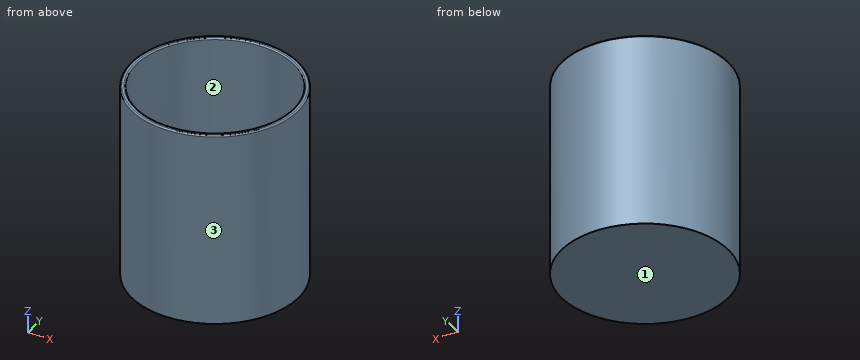
```python
from build123d import *

# Parameters (mm, degrees)
F0_R     = 30
F1_DEPTH = 70
F2_T     = -1.75
F3_R     = 0.5


with BuildPart() as f1:
    # F0 (on Top) → F1 (new body)
    with BuildSketch(Plane.XY):
        Circle(F0_R)
    extrude(amount=F1_DEPTH)

    # F2
    f2_openings = [f1.faces().sort_by_distance(p)[0] for p in [
        (0, 0, 70),
    ]]
    offset(amount=F2_T, openings=f2_openings)

    # F3
    f3_edges = [f1.edges().sort_by_distance(p)[0] for p in [
        (-30, 0, 70),
        (-28.25, 0, 70),
    ]]
    fillet(f3_edges, radius=F3_R)


solid = f1.part
```
CAD build for the part. Positions are in the model's coordinates, mm. Face numbers are marked on the shaded views. Round coordinates to 2 decimals unless told otherwise and drop trailing zeros. Loops run counter-clockwise (first coordinate to the right, second up) from the corner with the lowest first, then second, coordinate; pieces in that order, holes last. Notation, with made-up numbers: M -10,73.25 L 8,73.25 A17 ccw 8,100.25 Z; hole C 65,44 d4. An arc over 180 degrees is marked long. Use a Markdown table: item, result. Add a question column.
(1) Cut at A-A (z = 23). Give the cut face in (x, y).
(2) Flat gauge pins, fed straight in: pin 1 (1 mm diameter, centred on x = 11.5, z = 9.5, fed in from -Y); pin 2 (17 mm diameter, centred on x = 3, y = -5, fed in from +Z); pin 3 (3 mm diameter, centred on x = -16.5, z = 20.5, fed in from +Y). Where does each tip first touch, or does it go through?
(3) Drill centre lines: line 1 (Y direction, x = 0, z = 47.5); line 2 (X direction, y = -1, z = 25.5); line 3 (X direction, y = 19, z = 19). Where is each one in solid material? Low to high.
(4) Pull direction Y, two halves, no side cores. Call the marked faces 1, 2 and 3: +Y half, -Y half, draft (parallel to the pull), parting line (faces both ways), or undercut.
(5) Cut at B-B (x = 0). Give the cut face in (y, z), and give its area (3 significant figures).
Geometry says:
| question | item | result |
|---|---|---|
| 1 | outline | C 0,0 d60; hole C 0,0 d56.5 |
| 2 | pin 1 | stops at y = -27.91 |
| 2 | pin 2 | stops at z = 1.75 |
| 2 | pin 3 | stops at y = 25.98 |
| 3 | line 1 | y = -30 to -28.25, 28.25 to 30 |
| 3 | line 2 | x = -29.98 to -28.23, 28.23 to 29.98 |
| 3 | line 3 | x = -23.22 to -20.91, 20.91 to 23.22 |
| 4 | face 1 | draft |
| 4 | face 2 | undercut |
| 4 | face 3 | parting line |
| 5 | outline | M -30,0 L 30,0 L 30,69.5 A0.5 ccw 29.5,70 L 28.75,70 A0.5 ccw 28.25,69.5 L 28.25,1.75 L -28.25,1.75 L -28.25,69.5 A0.5 ccw -28.75,70 L -29.5,70 A0.5 ccw -30,69.5 Z |
| 5 | area | 344 mm² |
